Geometry check sheet. Reference: the model listing, model coordinates, mm. A direction names the side the tool comes from. Round coordinates to 2 decimals unless told otherwise and drop trailing zeros. Write each loop counter-clockwise with the first axis right and the second up, starting at its lowest first coordinate (ties: lowest second). Pieces come first, ordered by that corner, then holes. Notation, with made-up numbers: (87, 29) -> (120, 29) arc R23 ccw to (120, 68) -> close; hole circle Ø7 at (-23.5, 15.5). An arc over 180 degrees is marked (long way). Put each result on its own line as item: value. Start each with the question number.
from build123d import *

# Parameters (mm, degrees)
SKETCH1_W           = 7.6
SKETCH1_H           = 7.6
BOSS_EXTRUDE1_DEPTH = 7
SKETCH2_W           = 6.6
SKETCH2_H           = 6.6
CUT_EXTRUDE1_DEPTH  = 6.5
FILLET2_R           = 0.5


with BuildPart() as part:
    # Sketch1 → Boss-Extrude1 (new body)
    with BuildSketch(Plane(origin=(0, 0, 0), x_dir=(1, 0, 0), z_dir=(0, 1, 0))):
        Rectangle(SKETCH1_W, SKETCH1_H)
    extrude(amount=BOSS_EXTRUDE1_DEPTH)

    # Sketch2 → Cut-Extrude1 (cut)
    with BuildSketch(Plane.XZ):
        Rectangle(SKETCH2_W, SKETCH2_H)
    extrude(amount=-CUT_EXTRUDE1_DEPTH, mode=Mode.SUBTRACT)

    # Fillet2
    fillet2_edges = [part.edges().sort_by_distance(p)[0] for p in [
        (-3.8, 7, 0),
        (0, 7, 3.8),
        (0, 6.5, 3.3),
        (-3.3, 3.25, 3.3),
        (3.3, 6.5, 0),
        (3.3, 3.25, 3.3),
        (0, 6.5, -3.3),
        (3.3, 3.25, -3.3),
        (-3.3, 6.5, 0),
        (-3.3, 3.25, -3.3),
        (3.8, 7, 0),
        (0, 7, -3.8),
        (3.8, 3.5, 3.8),
        (-3.8, 3.5, 3.8),
        (-3.8, 3.5, -3.8),
        (3.8, 3.5, -3.8),
    ]]
    fillet(fillet2_edges, radius=FILLET2_R)


solid = part.part
(1) Mould release check, pull along X, two halves, no side actions. Record for faces 1 (the flat face through (0, 3, -3.8)), 2 (the flat face through (0, 3, 3.3)), 3 (the flat face through (3.8, 3, 0)): +X half, -X half, draft (parallel to the pull), parting line (faces both ways), or undercut.
(2) Set-up check for faces 4 (the flat face through (0, 6.5, 0)), 5 (the flat face through (-3.8, 3, 0)): record each of +Z, -Z, +X, -X, +Y, -Y from which the full face is reachable in a straight line by a thin tool's end or side.
(3) Sectioned sample at C-C (z = -2.25). Record the cut outline in (x, y), and give its area (3 significant figures).
(4) Sectioned sample at B-B (x = 1). Record the cut outline in (y, z).
(5) Go/stop test with a flat-tipped pin: pin 1 Ø1.7 at (x, z) = (-1, 0) entering from -Y. Record where the tip stops, or that it passes through.
(6) Sectioned sample at A-A (y = 0.5). Record the cut outline in (x, z).
(7) Material ranges on L1, parallel to X at y = 5, z = 0.75; L2, parallel to Y at x = -0.75, z = -1.5, recorded low to high. Write a range as from..to.
Found:
1. face 1: draft
1. face 2: undercut
1. face 3: +X half
2. face 4: -Y
2. face 5: +Z, -Z, -X, +Y, -Y
3. outline: (-3.8, 0) -> (-3.3, 0) -> (-3.3, 6) arc R0.5 cw to (-2.8, 6.5) -> (2.8, 6.5) arc R0.5 cw to (3.3, 6) -> (3.3, 0) -> (3.8, 0) -> (3.8, 6.5) arc R0.5 ccw to (3.3, 7) -> (-3.3, 7) arc R0.5 ccw to (-3.8, 6.5) -> close
3. area: 10.3 mm2
4. outline: (0, -3.8) -> (6.5, -3.8) arc R0.5 ccw to (7, -3.3) -> (7, 3.3) arc R0.5 ccw to (6.5, 3.8) -> (0, 3.8) -> (0, 3.3) -> (6, 3.3) arc R0.5 cw to (6.5, 2.8) -> (6.5, -2.8) arc R0.5 cw to (6, -3.3) -> (0, -3.3) -> close
5. pin 1: y = 6.5
6. outline: (-3.8, -3.3) arc R0.5 ccw to (-3.3, -3.8) -> (3.3, -3.8) arc R0.5 ccw to (3.8, -3.3) -> (3.8, 3.3) arc R0.5 ccw to (3.3, 3.8) -> (-3.3, 3.8) arc R0.5 ccw to (-3.8, 3.3) -> close; hole (-3.3, -2.8) arc R0.5 ccw to (-2.8, -3.3) -> (2.8, -3.3) arc R0.5 ccw to (3.3, -2.8) -> (3.3, 2.8) arc R0.5 ccw to (2.8, 3.3) -> (-2.8, 3.3) arc R0.5 ccw to (-3.3, 2.8) -> close
7. L1: -3.8..-3.3, 3.3..3.8
7. L2: 6.5..7
